Work out the finished part from the listing and answer in its coordinate system (mm). Face numbers are marked on the shaded views. Round coordinates to 2 decimals unless told otherwise and drop trailing zeros. Order: outer loops, then holes, each group sorted by start corner. A loop starts at its lowest first (then second) coordinate and runs counter-clockwise, first axis right, second up. Notation, with made-up numbers: (62.25, -10) - (113.25, -10) arc R11 ccw to (113.25, -4) - close; hole circle Ø9 at (-29, -34). An arc over 180 degrees is marked (long way). Put each result on its own line as item: value.
```python
from build123d import *
from build123d.topology import SkipClean

# Parameters (mm, degrees)
CROQUIS1_W                = 1.742923262
CROQUIS1_H                = 57.241679132
SALIENTE_EXTRUIR1_DEPTH   = 55
CROQUIS1_W_2              = 1.671507147
CROQUIS1_H_2              = 21.456626134
SALIENTE_EXTRUIR1_2_DEPTH = 55
CROQUIS2_W                = 3.684913484
CROQUIS2_H                = 21.456626134
SALIENTE_EXTRUIR2_DEPTH   = 2
CROQUIS3_W                = 6.689505602
CROQUIS3_H                = 21.456626134
SALIENTE_EXTRUIR3_DEPTH   = 1.742923
REDONDEO1_R               = 10
SALIENTE_EXTRUIR4_DEPTH   = 57


with BuildPart() as part:
    # Croquis1 → Saliente-Extruir1 (new body)
    with BuildSketch(Plane.XY):
        with Locations((-2.447737274, 25.2)):
            Rectangle(CROQUIS1_W, CROQUIS1_H)
    extrude(amount=-SALIENTE_EXTRUIR1_DEPTH)



with BuildPart() as body_2:
    # Croquis1 → Saliente-Extruir1 2 (new body)
    with BuildSketch(Plane.XY):
        with Locations((-6.168358816, 25.2)):
            Rectangle(CROQUIS1_W_2, CROQUIS1_H_2)
    extrude(amount=-SALIENTE_EXTRUIR1_2_DEPTH)


with BuildPart() as part_1:
    add(part.part)

    add(body_2.part)  # Saliente-Extruir2 merges body 2
    # Croquis2 → Saliente-Extruir2 (add)
    with BuildSketch(Plane.XY):
        with Locations((-5.161655647, 25.2)):
            Rectangle(CROQUIS2_W, CROQUIS2_H)
        Polygon((-3.319198905, 53.820839566), (-3.319198905, 35.928313067), (-3.319198905, 14.471686933), (-3.319198905, -3.420839566), (-1.576275643, -3.420839566), (-1.576275643, 14.471686933), (-1.576275643, 35.928313067), (-1.576275643, 53.820839566), align=None)
    extrude(amount=SALIENTE_EXTRUIR2_DEPTH)

    # Croquis3 → Saliente-Extruir3 (add, through all)
    with SkipClean():  # the faces are left unmerged after this step: merging them gives an invalid solid
        with BuildSketch(Plane.ZY.offset(3.319198905)):
            with Locations((-58.344752801, 25.2)):
                Rectangle(CROQUIS3_W, CROQUIS3_H)
        extrude(amount=-SALIENTE_EXTRUIR3_DEPTH)

    # Redondeo1
    # the kernel refuses this fillet: 10 mm, written as the material it takes off along each edge
    with BuildSketch(Plane(origin=(-26.909534167, 14.471686933, -61.689505602), x_dir=(0, 0, 1), z_dir=(1, 0, 0))) as redondeo1_piece_1:
        with BuildLine():
            CenterArc((10, -9.436134105), REDONDEO1_R, 109.332484587, 70.667515413)
            Line((0, -9.436134105), (-0.2, -9.436134105))
            Line((-0.2, -9.436134105), (-0.2, 0))
            Line((-0.2, 0), (0, 0.2))
            ThreePointArc((0, 0.2), (3.344752801, 0.2), (6.623295714, 0.188722682))
            Line((6.623295714, 0.188722682), (6.689505602, 0))
        make_face()
    extrude(amount=48.923593524, mode=Mode.SUBTRACT)
    with BuildSketch(Plane(origin=(-26.909534167, 35.928313067, -61.689505602), x_dir=(0, -1, 0), z_dir=(1, 0, 0))) as redondeo1_piece_2:
        with BuildLine():
            CenterArc((9.436134105, -10), REDONDEO1_R, 90, 70.667515413)
            Line((0, -6.689505602), (-0.188722682, -6.623295714))
            ThreePointArc((-0.188722682, -6.623295714), (-0.2, -3.344752801), (-0.2, 0))
            Line((-0.2, 0), (0, 0.2))
            Line((0, 0.2), (9.436134105, 0.2))
            Line((9.436134105, 0.2), (9.436134105, 0))
        make_face()
    extrude(amount=48.923593524, mode=Mode.SUBTRACT)

    # Croquis6 → Cortar-Revolución4 (revolve, cut)
    with SkipClean():  # the faces are left unmerged after this step: merging them gives an invalid solid
        with BuildSketch(Plane.ZY.offset(4.319198905)):
            with BuildLine():
                Line((-58.022003986, 30.9962324), (-58.022003986, 19.291046994))
                add(Edge.make_bspline(
                    [(-58.022003986, 30.9962324), (-60.287786898, 30.9962324), (-60.287786898, 25.143639697), (-60.287786898, 19.291046994), (-58.022003986, 19.291046994)],
                    knots=[3.141592654, 3.141592654, 3.141592654, 4.71238898, 4.71238898, 6.283185307, 6.283185307, 6.283185307], degree=2, weights=[1, 0.707106781, 1, 0.707106781, 1]))
            make_face()
        revolve(axis=Axis((-4.319198905, 19.291046994, -58.022003986), (0, 1, 0)), mode=Mode.SUBTRACT)

    # Croquis7 → Saliente-Extruir4 (add)
    with SkipClean():  # the faces are left unmerged after this step: merging them gives an invalid solid
        with BuildSketch(Plane(origin=(0, 0, -55), x_dir=(-1, 0, 0), z_dir=(0, 0, -1))):
            with BuildLine():
                Line((6.325110646, 50.074635433), (6.325110646, 49.12294906))
                Line((6.325110646, 49.12294906), (3.319198905, 49.12294906))
                Line((3.319198905, 49.12294906), (3.319198905, 53.820839566))
                Line((3.319198905, 53.820839566), (6.325110646, 53.820839566))
                Line((6.325110646, 53.820839566), (6.325110646, 52.869153193))
                ThreePointArc((6.325110646, 52.869153193), (4.927851766, 51.471894313), (6.325110646, 50.074635433))
            make_face()
            with BuildLine():
                Line((6.325110646, -3.420839566), (6.325110646, -2.469153193))
                ThreePointArc((6.325110646, -2.469153193), (4.927851766, -1.071894313), (6.325110646, 0.325364567))
                Line((6.325110646, 0.325364567), (6.325110646, 1.27705094))
                Line((6.325110646, 1.27705094), (3.319198905, 1.27705094))
                Line((3.319198905, 1.27705094), (3.319198905, -3.420839566))
                Line((3.319198905, -3.420839566), (6.325110646, -3.420839566))
            make_face()
        extrude(amount=-SALIENTE_EXTRUIR4_DEPTH)


solid = part_1.part
```
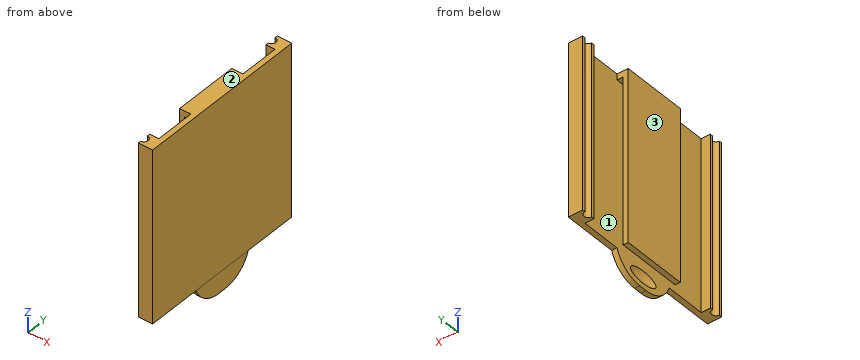
1) A cutting plane is placed at A-A on x = -4.1. Write down the section's boundary in (y, z), then the cut area to 3 significant figures.
Findings below:
outline: (-3.42, -55) - (1.28, -55) - (1.28, 2) - (-3.42, 2) - close; (14.47, 0) - (35.93, 0) - (35.93, 2) - (14.47, 2) - close; (49.12, -55) - (53.82, -55) - (53.82, 2) - (49.12, 2) - close
area: 578 mm2
2) Straight lines are drawn through the part: L1, parallel to X at y = 26.5, z = -8.5; L2, parallel to Y at x = -5.55, z = -37.5; L3, parallel to Y at x = -5.9, z = -21. For each, find the intervals that lie inside material, in ascending order. Write a range as from..to.
Findings below:
L1: x = -7..-5.33, -3.32..-1.58
L2: y = -3.42..-2.23, 0.09..1.28, 14.47..35.93, 49.12..50.31, 52.63..53.82
L3: y = -3.42..-2.4, 0.26..1.28, 14.47..35.93, 49.12..50.14, 52.8..53.82
3) For a pull along X with two mould halves and no side action, classify the marked faces 1, 2 and 3 as pulls with the +X half, pulls with the -X half, needs draft (parallel to the pull), parting line crosses it, or undercut.
Findings below:
face 1: undercut
face 2: needs draft
face 3: pulls with the -X half
4) A cutting plane is placed at D-D on y = 44.5. Write down the section's boundary in (x, z), then the cut area to 3 significant figures.
Findings below:
outline: (-3.32, -55) - (-1.58, -55) - (-1.58, 2) - (-3.32, 2) - close
area: 99.3 mm2
5) A cutting plane is placed at B-B on z = -19.5. Write down the section's boundary in (x, y), then the cut area to 3 significant figures.
Findings below:
outline: (-7, 14.47) - (-5.33, 14.47) - (-5.33, 35.93) - (-7, 35.93) - close; (-6.33, -3.42) - (-1.58, -3.42) - (-1.58, 53.82) - (-6.33, 53.82) - (-6.33, 52.87) arc R1.4 cw to (-6.33, 50.07) - (-6.33, 49.12) - (-3.32, 49.12) - (-3.32, 1.28) - (-6.33, 1.28) - (-6.33, 0.33) arc R1.4 cw to (-6.33, -2.47) - close
area: 158 mm2
6) Given pin 1 Ø0.5 at (y, z) = (53.5, -19.5) entering from -X; pin 2 Ø0.6 at (x, y) = (-5, 21) entering from -Z; pin 3 Ø1.8 at (x, y) = (-6, 24.5) entering from -Z, each flat-ended and moving along its own axis, determine where each tip first touches the part or whether it passes through.
Findings below:
pin 1: stops at x = -6.33
pin 2: stops at z = 0
pin 3: stops at z = -55
7) A cutting plane is placed at C-C on y = 35. Write down the section's boundary in (x, z).
Findings below:
outline: (-7, -55) - (-5.33, -55) - (-5.33, 0) - (-3.32, 0) - (-3.32, -56.94) - (-1.58, -56.94) - (-1.58, 2) - (-7, 2) - close
